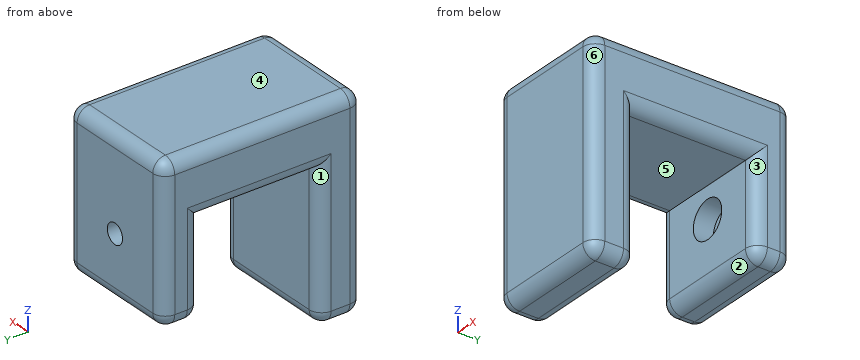
from build123d import *

# Parameters (mm, degrees)
F1_DEPTH       = 20
F3_D           = 3.2
F3_DEPTH       = 10
F3_CBORE_D     = 6
F3_CBORE_DEPTH = 3.2
F4_R           = 2


with BuildPart() as f1:
    # F0 (on Right) → F1 (new body)
    with BuildSketch(Plane.YZ):
        Polygon((6, 0), (0, 0), (-26, 0), (-26, -32.884616), (-19, -32.884616), (-19, -9.615385), (0, -9.615385), (0, -24.615385), (6, -24.615385), align=None)
    extrude(amount=F1_DEPTH)

    # F3
    with Locations(Plane.XZ):
        with Locations((10, -14.615385)):
            CounterBoreHole(F3_D / 2, F3_CBORE_D / 2, F3_CBORE_DEPTH, depth=F3_DEPTH)

    # F4
    f4_edges = [f1.edges().sort_by_distance(p)[0] for p in [
        (10, -26, 0),
        (20, -26, -16.442308),
        (20, -10, 0),
        (10, -26, -32.884616),
        (10, -19, -32.884616),
        (0, -22.5, -32.884616),
        (20, -22.5, -32.884616),
        (20, -19, -21.250001),
        (20, -9.5, -9.615385),
        (20, 0, -17.115385),
        (20, 3, -24.615385),
        (20, 6, -12.307692),
        (10, 0, -24.615385),
        (10, 6, -24.615385),
        (0, 3, -24.615385),
        (0, -10, 0),
        (0, -26, -16.442308),
        (0, -19, -21.250001),
        (0, -9.5, -9.615385),
        (0, 0, -17.115385),
        (0, 6, -12.307692),
        (10, 6, 0),
    ]]
    fillet(f4_edges, radius=F4_R)


solid = f1.part
Input: part model. Units: mm. Frame: model coordinates. Face numbers are marked on the shaded views. A direction names the side the tool comes from. Coordinates: 2 decimals unless noted, no trailing zeros. Order: outer loops, then holes, each group sorted by start corner. A loop starts at its lowest first (then second) coordinate and runs counter-clockwise, first axis right, second up.
1. Draft query along Y for the marked faces 4, 5 and 6. Return one class per face: +Y half, -Y half, draft (parallel to the pull), parting line (faces both ways), or undercut.
Checked values:
face 4: draft
face 5: undercut
face 6: -Y half
2. Cut plane C-C, the plane z = -30. Return loops of the section in (x, y), plus the area to 3 significant figures.
Checked values:
outline: (0, -24) arc R2 ccw to (2, -26) - (18, -26) arc R2 ccw to (20, -24) - (20, -21) arc R2 ccw to (18, -19) - (2, -19) arc R2 ccw to (0, -21) - close
area: 137 mm2
3. Access query for the marked faces 1, 2 and 3. Directions: +Z, -Z, +X, -X, +Y, -Y. A direction counts if a zero-diameter tool reaches every point of the face in a straight line with its end or side. Return the directions, or none.
Checked values:
face 1: -Z, -X
face 2: -Z, +X, -X
face 3: -Z, +X
4. Cut plane B-B, the plane y = -7.5. Return loops of the section in (x, z).
Checked values:
outline: (0, -7.62) arc R2 ccw to (2, -9.62) - (18, -9.62) arc R2 ccw to (20, -7.62) - (20, -2) arc R2 ccw to (18, 0) - (2, 0) arc R2 ccw to (0, -2) - close
5. Contact query for flat-ended pins moving along their axis: P1, Ø4, axis at x = 10, y = -16, coming from the -Z side; P2, Ø12, axis at y = -9.5, z = -19.5, coming from the +X side; P3, Ø1, axis at x = 9, y = 3, coming from the -Z side. Output: stop coordinate, or through.
Checked values:
P1: stops at z = -9.62
P2: passes through
P3: stops at z = -24.62
6. Ray query, line 1 along Y through (x, z) = (2, -11); line 2 along Z through (x, y) = (10, 4.1); line 3 along Z through (x, y) = (10, 2.5). Return the intervals inside material, ascending.
Checked values:
line 1: y = -26 to -19, 0 to 6
line 2: z = -24.61 to -16.22, -13.02 to 0
line 3: z = -24.62 to -17.62, -11.62 to 0
7. Cut plane A-A, the plane x = 10. Return loops of the section in (y, z), plus the area to 3 significant figures.
Checked values:
outline: (-26, -30.88) arc R2 ccw to (-24, -32.88) - (-21, -32.88) arc R2 ccw to (-19, -30.88) - (-19, -9.62) - (0, -9.62) - (0, -11.62) - (3.2, -11.62) - (3.2, -13.02) - (6, -13.02) - (6, -2) arc R2 ccw to (4, 0) - (-24, 0) arc R2 ccw to (-26, -2) - close; (0, -22.62) arc R2 ccw to (2, -24.62) - (4, -24.62) arc R2 ccw to (6, -22.62) - (6, -16.22) - (3.2, -16.22) - (3.2, -17.62) - (0, -17.62) - close
area: 527 mm2
